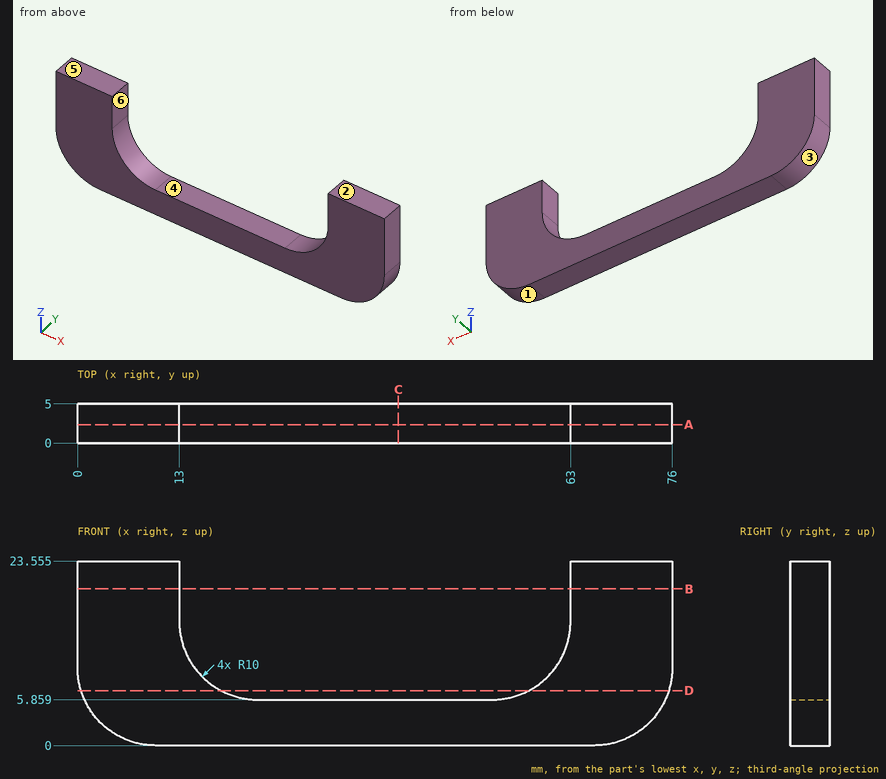
Geometry check sheet. Reference: drawing and pictorial views, mm from the part's lowest x, y, z. A direction names the side the tool comes from. Round coordinates to 2 decimals unless told otherwise and drop trailing zeros. Order: outer loops, then holes, each group sorted by start corner. A loop starts at its lowest first (then second) coordinate and runs counter-clockwise, first axis right, second up. Notation, with made-up numbers: M -17,25 L 25,25 A7 ccw 25,30 Z; hole C 47,86.5 d10. An arc over 180 degrees is marked long. Answer in a Markdown table with one row per item.
(1) Sectioned sample at C-C, the plane x = 41. Record the cut outline in (y, z).
Responses:
| item | result |
|---|---|
| outline | M 0,0 L 5,0 L 5,5.86 L 0,5.86 Z |
(2) Go/stop test with flat-tipped pins: P1, Ø4, axis at x = 59.5, z = 19.5, coming from the +Y side; P2, Ø2, axis at x = 53.5, y = 1.5, coming from the +Z side; P3, Ø1.5, axis at y = 4.5, z = 6.5, coming from the +X side; P4, Ø1.5, axis at x = 34, y = 2.5, coming from the +Z side. Record where each tip stops, or that it passes through.
Responses:
| item | result |
|---|---|
| P1 | passes through |
| P2 | stops at z = 5.97 |
| P3 | stops at x = 75.61 |
| P4 | stops at z = 5.86 |
(3) Sectioned sample at D-D, the plane z = 7. Record the cut outline in (x, y), and give its area (3 significant figures).
Responses:
| item | result |
|---|---|
| outline | M 0.46,0 L 18.36,0 L 18.36,5 L 0.46,5 Z; M 57.64,0 L 75.54,0 L 75.54,5 L 57.64,5 Z |
| area | 179 mm² |
(4) Sectioned sample at B-B, the plane z = 20. Record the cut outline in (x, y).
Responses:
| item | result |
|---|---|
| outline | M 0,0 L 13,0 L 13,5 L 0,5 Z; M 63,0 L 76,0 L 76,5 L 63,5 Z |
(5) Scan lines: probe 1 along X at (y, z) = (0.4, 16.5); probe 2 along Z at (x, y) = (49.5, 3.65); probe 3 along X at (y, z) = (1.1, 14.25). Record each from-to range of solid material in increasing order. Write a range as from..to.
Responses:
| item | result |
|---|---|
| probe 1 | x = 0..13, 63..76 |
| probe 2 | z = 0..5.86 |
| probe 3 | x = 0..13.13, 62.87..76 |
(6) Tool access check on the marked faces 5 and 6. Record the directions out of +Z, -Z, +X, -X, +Y, -Y that give a thin tool (end or side, any length) a straight path to the whole face; none if there is none.
Responses:
| item | result |
|---|---|
| face 5 | +Z, +X, -X, +Y, -Y |
| face 6 | +Z, +Y, -Y |
(7) Sectioned sample at A-A, the plane y = 2.35. Record the cut outline in (x, z) (1 decimal), and give its area (3 significant figures).
Responses:
| item | result |
|---|---|
| outline | M 0,10 A10 ccw 10,0 L 66,0 A10 ccw 76,10 L 76,23.6 L 63,23.6 L 63,15.9 A10 cw 53,5.9 L 23,5.9 A10 cw 13,15.9 L 13,23.6 L 0,23.6 Z |
| area | 905 mm² |
(8) Draft check along X on the marked faces 1, 2, 3 and 4. Enter one of: released by +X, released by -X, zero draft, split by the parting line, or undercut.
Responses:
| item | result |
|---|---|
| face 1 | released by +X |
| face 2 | zero draft |
| face 3 | released by -X |
| face 4 | undercut |
